Could you check a few things on this model? Use its own coordinates, in mm. A direction names the side the tool comes from. Round coordinates to 2 decimals unless told otherwise and drop trailing zeros. Loops run counter-clockwise (first coordinate to the right, second up) from the corner with the lowest first, then second, coordinate; pieces in that order, holes last. Notation, with made-up numbers: M 0,78 L 18,78 A17 ccw 18,86 Z; hole C -36.5,87 d3. An arc over 180 degrees is marked long. Answer in a Markdown table with one row per item.
```python
from build123d import *

# Parameters (mm, degrees)
SKETCH_1_W          = 120
SKETCH_1_H          = 15
EXTRUDE_1_DEPTH     = 5
SKETCH_2_R          = 1.6
CUT_EXTRUDE_1_DEPTH = 10
SKETCH_3_W          = 32
SKETCH_3_H          = 32
EXTRUDE_2_DEPTH     = 5
CUT_EXTRUDE_2_DEPTH = 7.5
FILLET_2_R          = 5
FILLET_4_R          = 5
CUT_EXTRUDE_3_DEPTH = 10
SKETCH_12_W         = 3.17
SKETCH_12_H         = 2
EXTRUDE_4_DEPTH     = 95


with BuildPart() as part:
    # Эскиз1 → Бобышка-Вытянуть1 (new body)
    with BuildSketch(Plane(origin=(0, 0, 0), x_dir=(1, 0, 0), z_dir=(0, 1, 0))):
        with Locations((-6.611570248, 6.549586777)):
            Rectangle(SKETCH_1_W, SKETCH_1_H)
    extrude(amount=EXTRUDE_1_DEPTH)

    # Эскиз2 → Вырез-Вытянуть1 (cut)
    with BuildSketch(Plane(origin=(0, 5, 0), x_dir=(1, 0, 0), z_dir=(0, 1, 0))):
        with Locations(Location((45.388429752, 6.549586777, 0), (0, 0, 270))):
            Circle(SKETCH_2_R)
        with Locations(Location((33.388429752, 6.549586777, 0), (0, 0, 270))):
            Circle(SKETCH_2_R)
    extrude(amount=-CUT_EXTRUDE_1_DEPTH, mode=Mode.SUBTRACT)

    # Эскиз3 → Бобышка-Вытянуть2 (add)
    with BuildSketch(Plane(origin=(0, 5, 0), x_dir=(1, 0, 0), z_dir=(0, 1, 0))):
        with Locations((-82.611570248, 6.549586777)):
            Rectangle(SKETCH_3_W, SKETCH_3_H)
    extrude(amount=-EXTRUDE_2_DEPTH)

    # Эскиз4 → Вырез-Вытянуть2 (cut)
    with BuildSketch(Plane(origin=(0, 5, 0), x_dir=(1, 0, 0), z_dir=(0, 1, 0))):
        with BuildLine():
            ThreePointArc((-95.412029446, 19.350045975), (-95.412029446, 17.087304275), (-93.149287746, 17.087304275))
            Line((-93.149287746, 17.087304275), (-95.412029446, 19.350045975))
        make_face()
        with BuildLine():
            Line((-95.412029446, 19.350045975), (-93.149287746, 17.087304275))
            ThreePointArc((-93.149287746, 17.087304275), (-92.802451344, 17.606381633), (-92.680658596, 18.218675125))
            ThreePointArc((-92.680658596, 18.218675125), (-93.668365104, 19.696882377), (-95.412029446, 19.350045975))
        make_face()
        with BuildLine():
            ThreePointArc((-69.812937508, 19.348219516), (-72.075679208, 19.348219516), (-72.075679208, 17.085477817))
            Line((-72.075679208, 17.085477817), (-69.812937508, 19.348219516))
        make_face()
        with BuildLine():
            Line((-69.812937508, 19.348219516), (-72.075679208, 17.085477817))
            ThreePointArc((-72.075679208, 17.085477817), (-70.332014867, 16.738641414), (-69.344308358, 18.216848666))
            ThreePointArc((-69.344308358, 18.216848666), (-69.466101106, 18.829142158), (-69.812937508, 19.348219516))
        make_face()
        with BuildLine():
            ThreePointArc((-93.147461288, -3.986304263), (-95.410202987, -3.986304263), (-95.410202987, -6.249045963))
            Line((-95.410202987, -6.249045963), (-93.147461288, -3.986304263))
        make_face()
        with BuildLine():
            Line((-93.147461288, -3.986304263), (-95.410202987, -6.249045963))
            ThreePointArc((-95.410202987, -6.249045963), (-93.666538646, -6.595882365), (-92.678832138, -5.117675113))
            ThreePointArc((-92.678832138, -5.117675113), (-92.800624885, -4.505381621), (-93.147461288, -3.986304263))
        make_face()
        with BuildLine():
            ThreePointArc((-69.346134817, -5.115848654), (-70.333841325, -3.637641402), (-72.077505667, -3.984477805))
            Line((-72.077505667, -3.984477805), (-69.814763967, -6.247219504))
            ThreePointArc((-69.814763967, -6.247219504), (-69.467927565, -5.728142146), (-69.346134817, -5.115848654))
        make_face()
        with BuildLine():
            Line((-69.814763967, -6.247219504), (-72.077505667, -3.984477805))
            ThreePointArc((-72.077505667, -3.984477805), (-72.077505667, -6.247219504), (-69.814763967, -6.247219504))
        make_face()
    extrude(amount=-CUT_EXTRUDE_2_DEPTH, mode=Mode.SUBTRACT)

    # Скругление2
    fillet_2_edges = [part.edges().sort_by_distance(p)[0] for p in [
        (-66.611570248, 2.5, 0.950413223),
    ]]
    fillet(fillet_2_edges, radius=FILLET_2_R)

    # Скругление4
    fillet_4_edges = [part.edges().sort_by_distance(p)[0] for p in [
        (-66.611570248, 2.5, -14.049586777),
    ]]
    fillet(fillet_4_edges, radius=FILLET_4_R)

    # Эскиз6 → Вырез-Вытянуть3 (cut)
    with BuildSketch(Plane(origin=(0, 5, 0), x_dir=(1, 0, 0), z_dir=(0, 1, 0))):
        Polygon((-62.351737512, 2.219586777), (-57.351737512, 10.879840815), (-52.351737512, 2.219586777), align=None)
        Polygon((-47.351737512, 2.219586777), (-42.351737512, 10.879840815), (-37.351737512, 2.219586777), align=None)
        Polygon((-32.351737512, 2.219586777), (-27.351737512, 10.879840815), (-22.351737512, 2.219586777), align=None)
        Polygon((-17.351737512, 2.219586777), (-12.351737512, 10.879840815), (-7.351737512, 2.219586777), align=None)
        Polygon((-2.351737512, 2.219586777), (2.648262488, 10.879840815), (7.648262488, 2.219586777), align=None)
        Polygon((-54.851737512, 10.879840815), (-49.851737512, 2.219586777), (-44.851737512, 10.879840815), align=None)
        Polygon((-39.851737512, 10.879840815), (-34.851737512, 2.219586777), (-29.851737512, 10.879840815), align=None)
        Polygon((-24.851737512, 10.879840815), (-19.851737512, 2.219586777), (-14.851737512, 10.879840815), align=None)
        Polygon((-9.851737512, 10.879840815), (-4.851737512, 2.219586777), (0.148262488, 10.879840815), align=None)
        Polygon((5.148262488, 10.879840815), (10.148262488, 2.219586777), (15.148262488, 10.879840815), align=None)
    extrude(amount=-CUT_EXTRUDE_3_DEPTH, mode=Mode.SUBTRACT)

    # Эскиз12 → Бобышка-Вытянуть4 (add)
    with BuildSketch(Plane(origin=(23.388429752, 0, 0), x_dir=(0, 0, -1), z_dir=(1, 0, 0))):
        with Locations((0.634586777, 6)):
            Rectangle(SKETCH_12_W, SKETCH_12_H)
        with Locations((12.464586777, 6)):
            Rectangle(SKETCH_12_W, SKETCH_12_H)
    extrude(amount=-EXTRUDE_4_DEPTH)


solid = part.part
```
1) I want a section at B-B, the plane x = -88. Please give me the cut outline in (y, z), plus the area to 3 significant figures.
Computed:
| item | result |
|---|---|
| outline | M 0,-22.55 L 5,-22.55 L 5,9.45 L 0,9.45 Z |
| area | 160 mm² |
2) Will these pins go through, and if not, where does the flat tip stop? P1, Ø2, axis at y = 6.5, z = -1, coming from the -X side; P2, Ø4, axis at y = 1.5, z = 7.5, coming from the +X side; P3, Ø2, axis at x = -38.5, z = -8, coming from the +Y side.
Computed:
| item | result |
|---|---|
| P1 | stops at x = -71.61 |
| P2 | stops at x = -66.59 |
| P3 | stops at y = 5 |
3) I want a section at D-D, the plane x = 26. Please give me the cut outline in (y, z), plus the area to 3 significant figures.
Computed:
| item | result |
|---|---|
| outline | M 0,-14.05 L 5,-14.05 L 5,0.95 L 0,0.95 Z |
| area | 75.0 mm² |
4) I need wall thicknesses on line 1 (Z direction, x = -69, y = 5.5); line 2 (Z direction, x = 33.5, y = 2.75); line 3 (Z direction, x = -54.5, y = 2). Which ranges of each line are inside material? Lowest first, please.
Computed:
| item | result |
|---|---|
| line 1 | z = -14.05 to -10.88, -2.22 to 0.95 |
| line 2 | z = -14.05 to -8.15, -4.95 to 0.95 |
| line 3 | z = -14.05 to -10.88, -10.27 to -5.94, -2.22 to 0.95 |
5) Which directions (+Z, -Z, +X, -X, +Y, -Y) give clear straight access to the entire face, cutting with the end or side of a thin tool? Please do faces 1 (the face through (-1, 5, -7)), 2 (the face through (-22.387, 2.535, -6.61)), 3 (the face through (-23, 4, -2.22)).
Computed:
| item | result |
|---|---|
| face 1 | +X, -X, +Y |
| face 2 | +Y, -Y |
| face 3 | +Y |
6) I want a section at A-A, the plane z = -3.5. State how many separate pieces and enclosed holes the cut face has, plus the area to 3 significant figures.
Computed:
| item | result |
|---|---|
| separate pieces | 11 |
| enclosed holes | 0 |
| area | 510 mm² |
7) If we mould it in two halves opening along Z, with no side actions, what happens to faces 4 (the face through (-5, 3, -10.88)), 5 (the face through (-65.11, 2.54, -15.48)), 6 (the face through (-8, 3, 0.95))? For each: released by +Z, released by -Z, zero draft, split by the parting line, or undercut.
Computed:
| item | result |
|---|---|
| face 4 | undercut |
| face 5 | released by -Z |
| face 6 | released by +Z |
